Model file for the job. Use its own axes, mm. A direction names the side the tool comes from. Coordinates: 2 decimals unless noted, no trailing zeros. Write each loop counter-clockwise with the first axis right and the second up, starting at its lowest first coordinate (ties: lowest second). Pieces come first, ordered by that corner, then holes. Notation, with made-up numbers: (-8.5, -38.5) -> (30.5, -38.5) arc R12 ccw to (30.5, -16.5) -> close; hole circle Ø10 at (8, 40.5). An arc over 180 degrees is marked (long way). Write item = value, one per line. Start each with the question number.
from build123d import *
from build123d.topology import SkipClean

# Parameters (mm, degrees)
SKETCH1_R           = 4.365625
SKETCH1_R_2         = 1.5
SKETCH1_R_3         = 3.75
SKETCH1_R_4         = 1
BOSS_EXTRUDE1_DEPTH = 2
BOSS_EXTRUDE2_START = 1.5875
SKETCH2_R           = 3.697441577
SKETCH2_R_2         = 1
BOSS_EXTRUDE2_DEPTH = 1.5875
SKETCH3_W           = 10.440578203
SKETCH3_H           = 0.489894741
CUT_EXTRUDE1_DEPTH  = 27.994455117
CUT_EXTRUDE3_DEPTH  = 29.041350462
BOSS_EXTRUDE3_START = 1
SKETCH6_R           = 4.365625
SKETCH6_R_2         = 1.5
BOSS_EXTRUDE3_DEPTH = 1
SKETCH7_R           = 4.365625
SKETCH7_R_2         = 1.5
BOSS_EXTRUDE4_DEPTH = 5


with BuildPart() as part:
    # Sketch1 → Boss-Extrude1 (new body)
    # profile 1 of 3: a face of its own
    with BuildSketch(Plane(origin=(0, 0, 0), x_dir=(1, 0, 0), z_dir=(0, 1, 0))):
        with BuildLine():
            Line((3.343145751, 4.365625), (0, 4.365625))
            ThreePointArc((0, 4.365625), (3.086963042, 3.086963042), (4.365625, 0))
            ThreePointArc((4.365625, 0), (3.086963042, -3.086963042), (0, -4.365625))
            Line((0, -4.365625), (1.467794033, -4.365625))
            ThreePointArc((1.467794033, -4.365625), (2.998527762, -4.67010687), (4.296221157, -5.537197875))
            Line((4.296221157, -5.537197875), (9.570119263, -10.81109598))
            ThreePointArc((9.570119263, -10.81109598), (10.198536879, -11.627006165), (10.597804983, -12.576323346))
            Line((10.597804983, -12.576323346), (11.898392678, -17.293417078))
            ThreePointArc((11.898392678, -17.293417078), (14.516748696, -12.681561512), (19.128604262, -15.29991753))
            Line((19.128604262, -15.29991753), (17.301580945, -8.673497591))
            ThreePointArc((17.301580945, -8.673497591), (16.902312841, -7.724180409), (16.273895225, -6.908270225))
            Line((16.273895225, -6.908270225), (6.171572875, 3.194052125))
            ThreePointArc((6.171572875, 3.194052125), (4.87387948, 4.06114313), (3.343145751, 4.365625))
        make_face()
    # profile 2 of 3: a face of its own
    with BuildSketch(Plane(origin=(0, 0, 0), x_dir=(1, 0, 0), z_dir=(0, 1, 0))):
        Circle(SKETCH1_R)
        with Locations(Location((0, 0, 0), (0, 0, 270))):
            Circle(SKETCH1_R_2, mode=Mode.SUBTRACT)
    # profile 3 of 3: a face of its own
    with BuildSketch(Plane(origin=(0, 0, 0), x_dir=(1, 0, 0), z_dir=(0, 1, 0))):
        with Locations((15.51349847, -16.296667304)):
            Circle(SKETCH1_R_3)
        with Locations(Location((15.51349847, -16.296667304, 0), (0, 0, 270))):
            Circle(SKETCH1_R_4, mode=Mode.SUBTRACT)
    extrude(amount=BOSS_EXTRUDE1_DEPTH)

    # Sketch2 → Boss-Extrude2 (add)
    # profile 1 of 2: a face of its own
    with SkipClean():  # the faces are left unmerged after this step: merging them gives an invalid solid
        with BuildSketch(Plane.XZ.offset(BOSS_EXTRUDE2_START)):
            with BuildLine():
                ThreePointArc((14.766930457, 12.675381563), (14.284086567, 12.809602551), (13.823828401, 13.007884965))
                Line((13.823828401, 13.007884965), (12.351641282, 8.832220322))
                Line((12.351641282, 8.832220322), (4.20896111, 0.85370709))
                Line((4.20896111, 0.85370709), (4.908830924, 0.139436662))
                Line((4.908830924, 0.139436662), (13.217481616, 8.280574235))
                Line((13.217481616, 8.280574235), (14.766930457, 12.675381563))
            make_face()
        # profile 2 of 2: a face of its own
        with BuildSketch(Plane.XZ.offset(BOSS_EXTRUDE2_START)):
            with Locations((15.51349847, 16.296667304)):
                Circle(SKETCH2_R)
            with Locations(Location((15.51349847, 16.296667304, 0), (0, 0, 270))):
                Circle(SKETCH2_R_2, mode=Mode.SUBTRACT)
        extrude(amount=-BOSS_EXTRUDE2_DEPTH)

    # Sketch3 → Cut-Extrude1 (cut, through all)
    with SkipClean():  # the faces are left unmerged after this step: merging them gives an invalid solid
        with BuildSketch(Plane(origin=(9.159515606, 0, -3.229311271), x_dir=(-0.33250340190554584, 0, -0.9431020558355491), z_dir=(0.9431020558355491, 0, -0.33250340190554584))):
            with Locations((-6.983995086, -1.34255263)):
                Rectangle(SKETCH3_W, SKETCH3_H)
            Polygon((-12.204284187, -1.097605259), (-16.864233023, -1.5875), (-12.204284187, -1.5875), align=None)
        extrude(amount=-CUT_EXTRUDE1_DEPTH, mode=Mode.SUBTRACT)

    # Sketch5 → Cut-Extrude3 (cut, through all)
    with SkipClean():  # the faces are left unmerged after this step: merging them gives an invalid solid
        with BuildSketch(Plane(origin=(1.634858863, 0, -1.668497934), x_dir=(0.7142704274254688, 0, 0.6998698139693111), z_dir=(-0.6998698139693111, 0, 0.7142704274254688))):
            with BuildLine():
                Line((15.003816491, -1.122033372), (4.466951764, -0.046116385))
                add(Edge.make_bspline(
                    [(3.855909999, 0), (4.032985789, 0), (4.289562434, -0.028003199), (4.466951764, -0.046116385)],
                    knots=[0, 0, 0, 0, 1, 1, 1, 1], degree=3))
                Line((3.855909999, 0), (3.579570092, 0))
                Line((3.579570092, 0), (3.579570092, -1.146381057))
                Line((3.579570092, -1.146381057), (15.003816491, -1.122033372))
            make_face()
        extrude(amount=-CUT_EXTRUDE3_DEPTH, mode=Mode.SUBTRACT)

    # Sketch6 → Boss-Extrude3 (add)
    with SkipClean():  # the faces are left unmerged after this step: merging them gives an invalid solid
        with BuildSketch(Plane.XZ.offset(BOSS_EXTRUDE3_START)):
            with Locations(Location((0, 0, 0), (0, 0, 270))):
                Circle(SKETCH6_R)
            with Locations(Location((0, 0, 0), (0, 0, 270))):
                Circle(SKETCH6_R_2, mode=Mode.SUBTRACT)
        extrude(amount=-BOSS_EXTRUDE3_DEPTH)

    # Sketch7 → Boss-Extrude4 (add)
    with BuildSketch(Plane(origin=(0, 2, 0), x_dir=(1, 0, 0), z_dir=(0, 1, 0))):
        with Locations(Location((0, 0, 0), (0, 0, 90))):
            Circle(SKETCH7_R)
        with Locations(Location((0, 0, 0), (0, 0, 90))):
            Circle(SKETCH7_R_2, mode=Mode.SUBTRACT)
    extrude(amount=BOSS_EXTRUDE4_DEPTH)


solid = part.part
(1) 3-axis set-ups, long thin cutter, end or side, ignore diameter. For faces 1 (the face through (1, 1, 4.366)), 2 (the face through (13.1, -0.63, 10.95)), 3 (the face through (10.9, -0.43, 6.01)), 4 (the face through (16.91, 0.99, 7.74)), 5 (the face through (10.196, -0.32, 6.72)): which of +Z, -Z, +X, -X, +Y, -Y reach the whole face in a straight line?
(2) Saw through at C-C (z = 6.5). Give the cut face in (x, y).
(3) Mould opens along X. For faces 6 (the face through (4.894, 0.986, -4.053)), 7 (the face through (2, 1, -4.366)), 8 (the face through (16.431, 0.986, 19.933)), 9 (the face through (8.99, -0.59, 4.84)) say: released by +X, released by -X, zero draft, split by the parting line, or undercut.
(4) Saw through at D-D (y = 3.75). Give the cut face in (x, z).
(5) Drill centre lines: line 1 along Y through (x, z) = (13, 15); line 2 along Z through (x, y) = (-0.75, 3.25); line 3 along Z through (x, y) = (1.25, 5.25). Where is each one in solid material? Low to high.
(6) Saw through at B-B (z = -1). Give the cut face in (x, y).
(7) Saw through at A-A (x = -0.5). Give the cut face in (y, z), then the cut area to 3 significant figures.
(8) Drop flat-ended pins along their axis: pin 1 Ø1.5 at (x, z) = (4, -1) entering from -Y; pin 2 Ø2.5 at (x, z) = (15.51, 16.3) entering from -Y; pin 3 Ø1.6 at (x, y) = (1, 1) entering from +Z; pin 4 Ø2 at (y, z) = (0.5, 13.5) entering from -X. Give the stop position or say it passes through.
Returned:
q1.face_1 = +Z, -X, +Y, -Y
q1.face_2 = -X, -Y
q1.face_3 = -Z, +X, -Y
q1.face_4 = -Z, +X, +Y, -Y
q1.face_5 = -Y
q2.outline = (5.26, 0) -> (9.97, 0) -> (9.97, -0.78) -> (11.4, -0.89) -> (11.4, 0) -> (15.87, 0) -> (15.87, 2) -> (5.26, 2) -> close
q3.face_6 = released by +X
q3.face_7 = zero draft
q3.face_8 = split by the parting line
q3.face_9 = undercut
q4.outline = circle Ø8.73 at (0, 0); hole circle Ø3 at (0, 0)
q5.line_1 = -1.59 to 2
q5.line_2 = -4.3 to -1.3, 1.3 to 4.3
q5.line_3 = -4.18 to -0.83, 0.83 to 4.18
q6.outline = (-4.25, -1) -> (-1.12, -1) -> (-1.12, 7) -> (-4.25, 7) -> close; (1.12, -1) -> (4.25, -1) -> (4.25, 0) -> (8.37, 0) -> (8.37, 2) -> (4.25, 2) -> (4.25, 7) -> (1.12, 7) -> close
q7.outline = (-1, -4.34) -> (7, -4.34) -> (7, -1.41) -> (-1, -1.41) -> close; (-1, 1.41) -> (7, 1.41) -> (7, 4.34) -> (-1, 4.34) -> close
q7.area = 46.8 mm2
q8.pin_1 = -1
q8.pin_2 = -1.59
q8.pin_3 = 4.38
q8.pin_4 = 10.58
